The listing builds one solid part. Answer for the finished solid, in the listing's coordinates (mm). A direction names the side the tool comes from. Round coordinates to 2 decimals unless told otherwise and drop trailing zeros. Loops run counter-clockwise (first coordinate to the right, second up) from the corner with the lowest first, then second, coordinate; pieces in that order, holes last. Notation, with made-up numbers: (14.25, 43.5) -> (49.25, 43.5) arc R16 ccw to (49.25, 55.5) -> close; hole circle Ø1 at (41, 34.25). An arc over 180 degrees is marked (long way). One line per question, with ' | ' between items.
from build123d import *

# Parameters (mm, degrees)
SKETCH1_R               = 72.5
SKETCH1_R_2             = 70
BOSS_EXTRUDE4_DEPTH     = 16
BOSS_EXTRUDE5_DEPTH     = 50
SKETCH2_R               = 1
CUT_EXTRUDE1_DEPTH      = 115.072345465
SKETCH3_R               = 50
SKETCH3_R_2             = 47
BOSS_EXTRUDE6_DEPTH     = 50
SKETCH1_12_R            = 72.5
SKETCH1_12_R_2          = 70
BOSS_EXTRUDE7_DEPTH     = 72.5
BOSS_EXTRUDE8_DEPTH     = 26
SKETCH5_W               = 25
SKETCH5_H               = 25
CUT_EXTRUDE4_DEPTH      = 137.5
SKETCH7_R               = 2.75
SKETCH7_R_2             = 2.5
BOSS_EXTRUDE9_DEPTH     = 5
SKETCH12_W              = 40
SKETCH12_H              = 45
CUT_EXTRUDE5_DEPTH      = 180
BOSS_EXTRUDE11_START    = -49.596857296
BOSS_EXTRUDE11_DEPTH    = 49.596857296
SKETCH12_2_W            = 40
SKETCH12_2_H            = 45
CUT_EXTRUDE6_DEPTH      = 199.5
CUT_EXTRUDE7_DEPTH      = 136.410776564
CUT_EXTRUDE7_DEPTH_BACK = 136.410776564
SKETCH17_W              = 54.58952291
SKETCH17_H              = 5.845779458
CUT_EXTRUDE8_DEPTH      = 158.362345779
CUT_EXTRUDE8_DEPTH_BACK = 158.362345779
SKETCH22_W              = 10
SKETCH22_H              = 10
BOSS_EXTRUDE12_DEPTH    = 22.903142704
CUT_EXTRUDE9_DEPTH      = 144.988394911
CUT_EXTRUDE9_DEPTH_BACK = 144.988394911
SKETCH24_W              = 215.86755616
SKETCH24_H              = 61.868005926
BOSS_EXTRUDE13_DEPTH    = 5
SKETCH27_W              = 40.372489194
SKETCH27_H              = 5.878977483
CUT_EXTRUDE11_DEPTH     = 5


with BuildPart() as part:
    # Sketch1 → Boss-Extrude4 (new body)
    with BuildSketch(Plane(origin=(0, 0, 0), x_dir=(1, 0, 0), z_dir=(0, 1, 0))):
        with Locations(Location((0, 0, 0), (0, 0, 270))):
            Circle(SKETCH1_R)
        with Locations(Location((0, 0, 0), (0, 0, 270))):
            Circle(SKETCH1_R_2, mode=Mode.SUBTRACT)
    extrude(amount=BOSS_EXTRUDE4_DEPTH)

    # Sketch1<11> → Boss-Extrude5 (add)
    with BuildSketch(Plane(origin=(0, 0, 0), x_dir=(1, 0, 0), z_dir=(0, 1, 0))):
        Polygon((1.5, 69.983926726), (0, 70.992443901), (-1.5, 69.983926726), (-1.5, 4.616525306), (-39.921994536, 57.499863933), (-41.728311549, 57.434093588), (-42.349045519, 55.736508176), (-3.927050983, 2.853169549), (-66.095144057, 23.052807466), (-67.51782638, 21.937871638), (-67.02219504, 20.199637917), (-4.854101966, 0), (-67.02219504, -20.199637917), (-67.51782638, -21.937871638), (-66.095144057, -23.052807466), (-3.927050983, -2.853169549), (-42.349045519, -55.736508176), (-41.728311549, -57.434093588), (-39.921994536, -57.499863933), (-1.5, -4.616525306), (-1.5, -69.983926726), (0, -70.992443901), (1.5, -69.983926726), (1.5, -4.616525306), (39.921994536, -57.499863933), (41.728311549, -57.434093588), (42.349045519, -55.736508176), (3.927050983, -2.853169549), (66.095144057, -23.052807466), (67.51782638, -21.937871638), (67.02219504, -20.199637917), (4.854101966, 0), (67.02219504, 20.199637917), (67.51782638, 21.937871638), (66.095144057, 23.052807466), (3.927050983, 2.853169549), (42.349045519, 55.736508176), (41.728311549, 57.434093588), (39.921994536, 57.499863933), (1.5, 4.616525306), align=None)
    extrude(amount=BOSS_EXTRUDE5_DEPTH)

    # Sketch2 → Cut-Extrude1 (cut, through all)
    with BuildSketch(Plane.XZ):
        with Locations(Location((0, 0, 0), (0, 0, 270))):
            Circle(SKETCH2_R)
    extrude(amount=-CUT_EXTRUDE1_DEPTH, mode=Mode.SUBTRACT)

    # Sketch3 → Boss-Extrude6 (add)
    with BuildSketch(Plane.XZ):
        Circle(SKETCH3_R)
        Circle(SKETCH3_R_2, mode=Mode.SUBTRACT)
    extrude(amount=-BOSS_EXTRUDE6_DEPTH)

    # Sketch1<12> → Boss-Extrude7 (add)
    with BuildSketch(Plane(origin=(0, 0, 0), x_dir=(1, 0, 0), z_dir=(0, 1, 0))):
        with Locations(Location((0, 0, 0), (0, 0, 270))):
            Circle(SKETCH1_12_R)
        with Locations(Location((0, 0, 0), (0, 0, 91.227860685))):
            Circle(SKETCH1_12_R_2, mode=Mode.SUBTRACT)
    extrude(amount=BOSS_EXTRUDE7_DEPTH)

    # Sketch6 → Boss-Extrude8 (add)
    with BuildSketch(Plane(origin=(0, 72.5, 0), x_dir=(1, 0, 0), z_dir=(0, 1, 0))):
        Polygon((-12.5, -95.356236397), (12.5, -95.356236397), (17.5, -95.356236397), (17.5, -70.356236397), (12.5, -70.356236397), (-12.5, -70.356236397), (-17.5, -70.356236397), (-17.5, -95.356236397), align=None)
    extrude(amount=-BOSS_EXTRUDE8_DEPTH)

    # Sketch5 → Cut-Extrude4 (cut)
    with BuildSketch(Plane.XY):
        with Locations((0, 72.5)):
            Rectangle(SKETCH5_W, SKETCH5_H)
    extrude(amount=CUT_EXTRUDE4_DEPTH, mode=Mode.SUBTRACT)

    # Sketch7 → Boss-Extrude9 (add)
    # profile 1 of 2: a face of its own
    with BuildSketch(Plane(origin=(0, 72.5, 0), x_dir=(1, 0, 0), z_dir=(0, 1, 0))):
        with BuildLine():
            Line((-30, -82.856236397), (-30, -66.001893912))
            Line((-30, -66.001893912), (-17.5, -70.356236397))
            Line((-17.5, -70.356236397), (-17.5, -95.356236397))
            ThreePointArc((-17.5, -95.356236397), (-26.338834765, -91.695071162), (-30, -82.856236397))
        make_face()
        with Locations(Location((-23.75, -82.856236397, 0), (0, 0, 270))):
            Circle(SKETCH7_R, mode=Mode.SUBTRACT)
    # profile 2 of 2: a face of its own
    with BuildSketch(Plane(origin=(0, 72.5, 0), x_dir=(1, 0, 0), z_dir=(0, 1, 0))):
        with BuildLine():
            Line((30, -82.856236397), (30, -66.001893912))
            Line((30, -66.001893912), (17.5, -70.356236397))
            Line((17.5, -70.356236397), (17.5, -95.356236397))
            ThreePointArc((17.5, -95.356236397), (26.338834765, -91.695071162), (30, -82.856236397))
        make_face()
        with Locations(Location((23.75, -82.856236397, 0), (0, 0, 270))):
            Circle(SKETCH7_R_2, mode=Mode.SUBTRACT)
    extrude(amount=-BOSS_EXTRUDE9_DEPTH)

    # Sketch12 → Cut-Extrude5 (cut)
    with BuildSketch(Plane.XY):
        with Locations((0, 72.5)):
            Rectangle(SKETCH12_W, SKETCH12_H)
    extrude(amount=-CUT_EXTRUDE5_DEPTH, mode=Mode.SUBTRACT)

    # Sketch15 → Boss-Extrude11 (add)
    with BuildSketch(Plane(origin=(0, 72.5, 0), x_dir=(1, 0, 0), z_dir=(0, 1, 0)).offset(BOSS_EXTRUDE11_START)):
        with BuildLine():
            Line((-25, 103.053287944), (25, 103.053287944))
            Line((25, 103.053287944), (25, 68.053287944))
            ThreePointArc((25, 68.053287944), (0, 72.5), (-25, 68.053287944))
            Line((-25, 68.053287944), (-25, 103.053287944))
        make_face()
    extrude(amount=BOSS_EXTRUDE11_DEPTH)

    # Sketch12<2> → Cut-Extrude6 (cut)
    with BuildSketch(Plane.XY):
        with Locations((0, 72.5)):
            Rectangle(SKETCH12_2_W, SKETCH12_2_H)
    extrude(amount=-CUT_EXTRUDE6_DEPTH, mode=Mode.SUBTRACT)

    # Sketch17 → Cut-Extrude7 (cut, two sides: drawn at the far end of the back side and taken through both)
    with BuildSketch(Plane.XZ.offset(-22.903142704).offset(-CUT_EXTRUDE7_DEPTH_BACK)):
        with Locations((-0.620011984, -102.924929054)):
            Rectangle(SKETCH17_W, SKETCH17_H)
    extrude(amount=CUT_EXTRUDE7_DEPTH + CUT_EXTRUDE7_DEPTH_BACK, mode=Mode.SUBTRACT)

    # Sketch20 → Cut-Extrude8 (cut, two sides: drawn at the far end of the back side and taken through both)
    with BuildSketch(Plane(origin=(25, 0, 0), x_dir=(0, 0, -1), z_dir=(1, 0, 0)).offset(-CUT_EXTRUDE8_DEPTH_BACK)):
        with BuildLine():
            Line((83.502039325, 66.8), (86.502039325, 66.8))
            ThreePointArc((86.502039325, 66.8), (88.302039325, 65), (86.502039325, 63.2))
            Line((86.502039325, 63.2), (83.502039325, 63.2))
            ThreePointArc((83.502039325, 63.2), (81.702039325, 65), (83.502039325, 66.8))
        make_face()
    extrude(amount=CUT_EXTRUDE8_DEPTH + CUT_EXTRUDE8_DEPTH_BACK, mode=Mode.SUBTRACT)

    # Sketch22 → Boss-Extrude12 (add)
    with BuildSketch(Plane.XZ.offset(-22.903142704)):
        with Locations((0, -77.327380707)):
            Rectangle(SKETCH22_W, SKETCH22_H)
    extrude(amount=BOSS_EXTRUDE12_DEPTH)

    # Sketch24 → Cut-Extrude9 (cut, two sides: drawn at the far end of the back side and taken through both)
    with BuildSketch(Plane(origin=(1.5, 0, 0), x_dir=(0, 0, -1), z_dir=(1, 0, 0)).offset(-CUT_EXTRUDE9_DEPTH_BACK)):
        with Locations((14.738289666, 16.065997037)):
            Rectangle(SKETCH24_W, SKETCH24_H)
    extrude(amount=CUT_EXTRUDE9_DEPTH + CUT_EXTRUDE9_DEPTH_BACK, mode=Mode.SUBTRACT)

    # Sketch25 → Boss-Extrude13 (add)
    with BuildSketch(Plane(origin=(0, 50, 0), x_dir=(1, 0, 0), z_dir=(0, 1, 0))):
        with BuildLine():
            Line((-20, 67.082039325), (-20, 100.002039325))
            Line((-20, 100.002039325), (20, 100.002039325))
            Line((20, 100.002039325), (20, 67.082039325))
            ThreePointArc((20, 67.082039325), (0, 70), (-20, 67.082039325))
        make_face()
    extrude(amount=BOSS_EXTRUDE13_DEPTH)

    # Sketch27 → Cut-Extrude11 (cut)
    with BuildSketch(Plane(origin=(0, 0, 93.195488414), x_dir=(-1, 0, 0), z_dir=(0, 0, -1))):
        with Locations((1.632930754, 44.060511259)):
            Rectangle(SKETCH27_W, SKETCH27_H)
    extrude(amount=-CUT_EXTRUDE11_DEPTH, mode=Mode.SUBTRACT)


solid = part.part
Q1. A cutting plane is placed at B-B on x = -58. Give the vertices of the cut face in (y, z), plus the area to 3 significant figures.
Numbers:
outline: (47, -43.5) -> (72.5, -43.5) -> (72.5, -39.19) -> (47, -39.19) -> close; (47, -20.42) -> (50, -20.42) -> (50, -17.27) -> (47, -17.27) -> close; (47, 17.27) -> (50, 17.27) -> (50, 20.42) -> (47, 20.42) -> close; (47, 39.19) -> (72.5, 39.19) -> (72.5, 43.5) -> (47, 43.5) -> close | area: 239 mm^2
Q2. Find the intervals of material crossed by line 1 (X direction, y = 70, z = 75); line 2 (X direction, y = 48.75, z = 63); line 3 (X direction, y = 53.75, z = 0), in increasing order. Write a range as from..to.
Numbers:
line 1: -30..-12.5, 12.5..30 | line 2: -35.88..-30.51, -1.5..1.5, 30.51..35.88 | line 3: -72.5..-70, 70..72.5
Q3. For faces 4 (the face through (30, 70, 75)), 5 (the face through (-22, 67.5, 80)), 6 (the face through (25, 60, -84)), 7 (the face through (17.5, 57, 83)), 8 (the face through (57.375, 48.479, -17.065)), determine the directions among +Z, -Z, +X, -X, +Y, -Y from which every point of the face is accessible in a straight line to the end or side of a thin tool.
Numbers:
face 4: +Z, +X, +Y, -Y | face 5: +Z, -X, -Y | face 6: -Z, +X, +Y, -Y | face 7: +Z, +X, -Y | face 8: +Y, -Y
Q4. For a pull along X with two mould halves and no side action, classify faces 1 (the face through (26.241, 70.035, 91.792)), 2 (the face through (-14.123, 48.479, 21.991)), 3 (the face through (-26.241, 70.035, 91.792)) as pulls with the +X half, pulls with the -X half, needs draft (parallel to the pull), parting line crosses it, or undercut.
Numbers:
face 1: pulls with the +X half | face 2: undercut | face 3: pulls with the -X half
Q5. Given pin 1 Ø3.5 at (y, z) = (49, -32.5) entering from -X; pin 2 Ø6 at (y, z) = (63, 55) entering from +X; pin 3 Ø20 at (x, z) = (-0.5, 84.5) entering from +Y, each flat-ended and moving along its own axis, determine where each tip first touches the part or whether it passes through.
Numbers:
pin 1: x = -65.66 | pin 2: x = 50.52 | pin 3: y = 60
Q6. A cutting plane is placed at A-A on z = -43.5. Give the vertices of the cut face in (x, y), plus the area to 3 significant figures.
Numbers:
outline: (-58, 47) -> (-54.84, 47) -> (-54.84, 72.5) -> (-58, 72.5) -> close; (-33.46, 47) -> (-29.75, 47) -> (-29.75, 50) -> (-33.46, 50) -> close; (-24.65, 47) -> (-17.8, 47) -> (-17.8, 50) -> (-24.65, 50) -> close; (-1.5, 47) -> (1.5, 47) -> (1.5, 50) -> (-1.5, 50) -> close; (17.8, 47) -> (24.65, 47) -> (24.65, 50) -> (17.8, 50) -> close; (29.75, 47) -> (33.46, 47) -> (33.46, 50) -> (29.75, 50) -> close; (54.84, 47) -> (58, 47) -> (58, 72.5) -> (54.84, 72.5) -> close | area: 233 mm^2
